Read the model definition and answer for the solid it produces. Units are mm, in the model's axes. A direction names the side the tool comes from. Coordinates: 2 decimals unless noted, no trailing zeros. Order: outer loops, then holes, each group sorted by start corner. A loop starts at its lowest first (then second) coordinate and runs counter-clockwise, first axis right, second up. Notation, with made-up numbers: (39, 14.25) - (95, 14.25) arc R21 cw to (95, 31.25) - close; hole circle Ø9 at (-28.5, 85). An arc over 180 degrees is marked (long way). Write item = value, one per line.
from build123d import *

# Parameters (mm, degrees)
EXTRUSION1_DEPTH          = 10
TROU_TARAUD_M4X0_71_D     = 3.3
TROU_TARAUD_M4X0_71_DEPTH = 15
TROU_TARAUD_M4X0_71_TIP   = 0.991420021
ESQUISSE4_R               = 5
ENL_V_MAT_EXTRU_1_DEPTH   = 131.384048104
TROU_TARAUD_M31_D         = 2.5
ESQUISSE7_R               = 1.5
ENL_V_MAT_EXTRU_2_DEPTH   = 10


with BuildPart() as part:
    # Esquisse1 → Extrusion1 (new body)
    with BuildSketch(Plane.XY):
        with BuildLine():
            Line((-40, 9), (-50, 9))
            Line((-50, 9), (-50, 120))
            Line((-50, 120), (50, 120))
            Line((50, 120), (50, 9))
            Line((50, 9), (40, 9))
            Line((40, 9), (40, 60))
            ThreePointArc((40, 60), (38.535533906, 63.535533906), (35, 65))
            Line((35, 65), (-35, 65))
            ThreePointArc((-35, 65), (-38.535533906, 63.535533906), (-40, 60))
            Line((-40, 60), (-40, 9))
        make_face()
    extrude(amount=EXTRUSION1_DEPTH)

    # Trou taraudé M4x0.71
    with Locations(Plane.XZ.offset(-9)):
        with Locations((-45, 5), (45, 5)):
            Hole(TROU_TARAUD_M4X0_71_D / 2, depth=TROU_TARAUD_M4X0_71_DEPTH)
            with Locations((0, 0, -(TROU_TARAUD_M4X0_71_DEPTH + TROU_TARAUD_M4X0_71_TIP / 2))):  # 118° drill point
                Cone(0, TROU_TARAUD_M4X0_71_D / 2, TROU_TARAUD_M4X0_71_TIP, mode=Mode.SUBTRACT)

    # Esquisse4 → Enlèv. mat.-Extru.1 (cut, through all)
    with BuildSketch(Plane.XY):
        with Locations((14.5, 114)):
            Circle(ESQUISSE4_R)
        with Locations((-5.5, 114)):
            Circle(ESQUISSE4_R)
        with BuildLine():
            Line((22.25, 107), (13.25, 107))
            ThreePointArc((13.25, 107), (11.128679656, 106.121320344), (10.25, 104))
            Line((10.25, 104), (10.25, 95))
            ThreePointArc((10.25, 95), (11.128679656, 92.878679656), (13.25, 92))
            Line((13.25, 92), (22.25, 92))
            ThreePointArc((22.25, 92), (24.371320344, 92.878679656), (25.25, 95))
            Line((25.25, 95), (25.25, 104))
            ThreePointArc((25.25, 104), (24.371320344, 106.121320344), (22.25, 107))
        make_face()
    extrude(amount=ENL_V_MAT_EXTRU_1_DEPTH, mode=Mode.SUBTRACT)

    # Trou taraudé M31 (through all)
    with Locations(Plane(origin=(0, 0, 0), x_dir=(-1, 0, 0), z_dir=(0, 0, -1))):
        with Locations((-23.5, 112.5), (14.5, 112.5), (-20.5, 67), (-47, 117), (47, 117), (47, 33), (-47, 33)):
            Hole(TROU_TARAUD_M31_D / 2)

    # Esquisse7 → Enlèv. mat.-Extru.2 (cut)
    with BuildSketch(Plane(origin=(0, 120, 0), x_dir=(1, 0, 0), z_dir=(0, 1, 0))):
        with Locations(Location((35, -5, 0), (0, 0, 270))):
            Circle(ESQUISSE7_R)
    extrude(amount=-ENL_V_MAT_EXTRU_2_DEPTH, mode=Mode.SUBTRACT)


solid = part.part
1) Determine the mould class of faces 1 (the face through (18, 107, 5)), 2 (the face through (1, 78, 10)) for opening direction X: pulls with the +X half, pulls with the -X half, needs draft (parallel to the pull), parting line crosses it, or undercut.
Returned:
face_1 = undercut
face_2 = needs draft
2) Straight lines are drawn through the part: line 1 along Y through (x, z) = (-47, 4.25); line 2 along Y through (x, z) = (14.5, 3.25); line 3 along X through (y, z) = (19.5, 5). For each, find the intervals that lie inside material, in ascending order. Write a range as from..to.
Returned:
line_1 = 9..31.75, 34.25..115.75, 118.25..120
line_2 = 65..92, 107..109, 119..120
line_3 = -50..-46.65, -43.35..-40, 40..43.35, 46.65..50
3) The part is cut by section D-D (x = 14.5). Determine the outline of the cut face in (y, z).
Returned:
outline = (65, 0) - (92, 0) - (92, 10) - (65, 10) - close; (107, 0) - (109, 0) - (109, 10) - (107, 10) - close; (119, 0) - (120, 0) - (120, 10) - (119, 10) - close
4) Flat-ended cylindrical pins translate along their axes: pin 1 Ø3 at (x, y) = (-47, 33) entering from -Z; pin 2 Ø6 at (x, z) = (36, 5) entering from -Y; pin 3 Ø2.5 at (x, z) = (35, 5) entering from -Y. Find the tip coordinate at first contact, or state that the pin passes through.
Returned:
pin_1 = 0
pin_2 = 63
pin_3 = 64.84
5) The part is cut by section B-B (x = -5.5). Determine the outline of the cut face in (y, z), and give its area (3 significant figures).
Returned:
outline = (65, 0) - (109, 0) - (109, 10) - (65, 10) - close; (119, 0) - (120, 0) - (120, 10) - (119, 10) - close
area = 450 mm^2
6) For faces 3 (the face through (46.65, 16.6, 5.07)), 4 (the face through (40, 34, 5)), 5 (the face through (11.11, 92.9, 4.93)), determine the directions among +Z, -Z, +X, -X, +Y, -Y from which every point of the face is accessible in a straight line to the end or side of a thin tool.
Returned:
face_3 = -Y
face_4 = +Z, -Z, -Y
face_5 = +Z, -Z
7) The part is cut by section A-A (z = 1.25). Count the separate pieces of the cut face and the enclosed holes in it, and give its area (3 significant figures).
Returned:
separate_pieces = 1
enclosed_holes = 10
area = 6,220 mm^2
8) The part is cut by section C-C (y = 99). Determine the outline of the cut face in (x, z).
Returned:
outline = (-50, 0) - (10.25, 0) - (10.25, 10) - (-50, 10) - close; (25.25, 0) - (50, 0) - (50, 10) - (25.25, 10) - close
